```python
from build123d import *

# Parameters (mm, degrees)
EXTRUDE_THIN2_DEPTH = 60
SKETCH2_W           = 60
SKETCH2_H           = 60
BOSS_EXTRUDE1_DEPTH = 5
FILLET5_R           = 5
FILLET6_R           = 5
FILLET7_R           = 5
FILLET8_R           = 5


with BuildPart() as part:
    # Sketch1 → Extrude-Thin2 (new body)
    with BuildSketch(Plane.XY):
        Polygon((34.692024717, 0), (-25.307975283, 0), (-64.323670762, 69.841073204), (-55.593536612, 74.718035139), (-19.439751523, 10), (34.692024717, 10), align=None)
    extrude(amount=EXTRUDE_THIN2_DEPTH)

    # Sketch2 → Boss-Extrude1 (add)
    with BuildSketch(Plane.XZ):
        with Locations((4.692024717, 30)):
            Rectangle(SKETCH2_W, SKETCH2_H)
    extrude(amount=BOSS_EXTRUDE1_DEPTH)

    # Fillet5
    fillet5_edges = [part.edges().sort_by_distance(p)[0] for p in [
        (-59.958603687, 72.279554172, 60),
    ]]
    fillet(fillet5_edges, radius=FILLET5_R)

    # Fillet6
    fillet6_edges = [part.edges().sort_by_distance(p)[0] for p in [
        (34.692024717, 2.5, 60),
    ]]
    fillet(fillet6_edges, radius=FILLET6_R)

    # Fillet7
    fillet7_edges = [part.edges().sort_by_distance(p)[0] for p in [
        (34.692024717, 2.5, 0),
    ]]
    fillet(fillet7_edges, radius=FILLET7_R)

    # Fillet8
    fillet8_edges = [part.edges().sort_by_distance(p)[0] for p in [
        (-59.958603687, 72.279554172, 0),
    ]]
    fillet(fillet8_edges, radius=FILLET8_R)


solid = part.part
```
Geometry: final body of the model. Coordinates: model frame, mm. A direction names the side the tool comes from. Give positions to 0.01 mm unless a question says otherwise; leave off trailing zeros. Write each loop counter-clockwise with the first axis right and the second up, starting at its lowest first coordinate (ties: lowest second). Pieces come first, ordered by that corner, then holes.
1. Section query D-D, the plane x = -37. Return loops of the section in (y, z).
2. Section query A-A, the plane z = 23.5. Return loops of the section in (x, y).
3. Section query B-B, the plane x = 28. Return loops of the section in (y, z), then the cut area to 3 significant figures.
4. Line query: probe 1 along Y at (x, z) = (-16, 42.5); probe 2 along X at (y, z) = (9.5, 6.5); probe 3 along Y at (x, z) = (-24.5, 41). Output: solid intervals per line, ascending.
5. Reachability of faces 1 (the flat face through (7, 10, 30)), 2 (the flat face through (-25.308, -2, 30)), 3 (the cylindrical face through (33.19, 2.61, 58.57)) from +Z, -Z, +X, -X, +Y, -Y: full face, straight path, thin tool, end or side. Return the list, or none.
6. Pin query (flat end, axial travel): P1, Ø6, axis at y = 13.5, z = 15.5, coming from the -X side; P2, Ø3, axis at x = -42, y = 50.5, coming from the +Z side; P3, Ø6, axis at y = 6.5, z = 44, coming from the -X side (3 decimals); P4, Ø16, axis at x = 2, z = 16, coming from the +Y side. Return the tip coordinate at first contact, or that it passes through.
7. Section query C-C, the plane y = 8.5. Return loops of the section in (x, z), then the cut area to 3 significant figures.
Computed:
1. outline: (20.93, 0) - (41.43, 0) - (41.43, 60) - (20.93, 60) - close
2. outline: (-64.32, 69.84) - (-25.31, 0) - (-25.31, -5) - (34.69, -5) - (34.69, 10) - (-19.44, 10) - (-55.59, 74.72) - close
3. outline: (-5, 0) - (10, 0) - (10, 60) - (-5, 60) - close
3. area: 900 mm2
4. probe 1: y = -5 to 10
4. probe 2: x = -30.62 to 34.69
4. probe 3: y = -5 to 19.06
5. face 1: +Z, -Z, +X, +Y
5. face 2: +Z, -Z, -X, -Y
5. face 3: +Z, +X, +Y, -Y
6. P1: stops at x = -34.53
6. P2: stops at z = 60
6. P3: stops at x = -30.615
6. P4: stops at y = 10
7. outline: (-30.06, 0) - (29.69, 0) arc R5 ccw to (34.69, 5) - (34.69, 55) arc R5 ccw to (29.69, 60) - (-30.06, 60) - close
7. area: 3,870 mm2
